Drawing for the job (mm, zero at the part's lowest x, y, z). A direction names the side the tool comes from. Give positions to 0.01 mm unless a question says otherwise; leave off trailing zeros. Order: outer loops, then holes, each group sorted by start corner. A loop starts at its lowest first (then second) coordinate and runs counter-clockwise, first axis right, second up. Notation, with made-up numbers: M -8.75,-21.75 L 24.25,-21.75 A21 ccw 24.25,3.25 Z; hole C 2.25,-22 d8. An arc over 180 degrees is marked long. Answer as a JSON object with one key per item and string values.
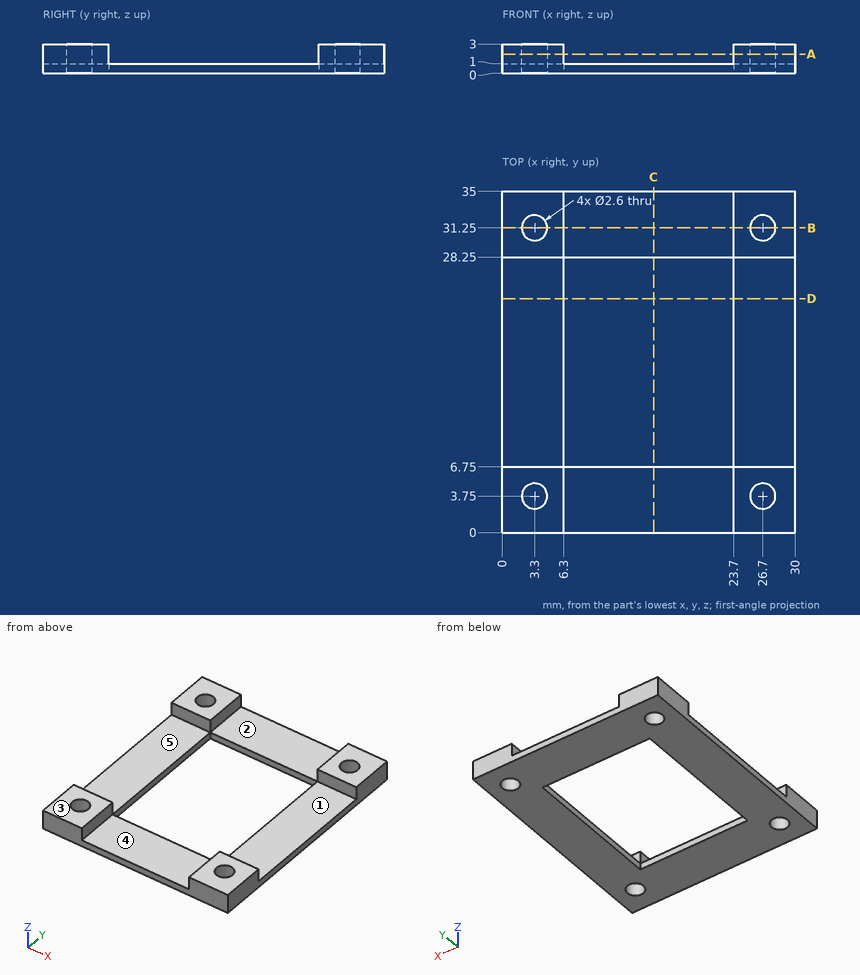
1. Pin check, flat tips, straight feed: P1, Ø4, axis at x = 5, y = 11.5, coming from the +Z side; P2, Ø2.5, axis at x = 3.3, y = 31.25, coming from the -Z side; P3, Ø1.1, axis at x = 11.5, z = 0.5, coming from the -Y side. Stop position of each tip, or through.
Worked answers:
{"P1": "stops at z = 1", "P2": "passes through", "P3": "stops at y = 0"}
2. Which spindle directions (+Z, -Z, +X, -X, +Y, -Y) get a long thin tool onto all of the face, cutting with end or side? Do the marked faces 1, 2 and 3. Say none if no direction does.
Worked answers:
{"face 1": "+Z, +X, -X", "face 2": "+Z, +Y, -Y", "face 3": "+Z, +X, -X, +Y, -Y"}
3. Cut at A-A on z = 1.95. Give the cut face in (x, y), plus the area to 3 significant figures.
Worked answers:
{"outline": "M 0,0 L 6.3,0 L 6.3,6.75 L 0,6.75 Z; M 0,28.25 L 6.3,28.25 L 6.3,35 L 0,35 Z; M 23.7,0 L 30,0 L 30,6.75 L 23.7,6.75 Z; M 23.7,28.25 L 30,28.25 L 30,35 L 23.7,35 Z; hole C 3.3,3.75 d2.6; hole C 3.3,31.25 d2.6; hole C 26.7,3.75 d2.6; hole C 26.7,31.25 d2.6", "area": "149 mm^2"}
4. Cut at B-B on y = 31.25. Give the cut face in (x, z), plus the area to 3 significant figures.
Worked answers:
{"outline": "M 0,0 L 2,0 L 2,3 L 0,3 Z; M 4.6,0 L 25.4,0 L 25.4,3 L 23.7,3 L 23.7,1 L 6.3,1 L 6.3,3 L 4.6,3 Z; M 28,0 L 30,0 L 30,3 L 28,3 Z", "area": "39.6 mm^2"}
5. Two-plate mould, pull along X, no slides. Class the marked faces 4 and 5: +X half, -X half, draft (parallel to the pull), parting line (faces both ways), or undercut.
Worked answers:
{"face 4": "undercut", "face 5": "draft"}
6. Probe line 1 along Y through (x, z) = (26.7, 0.85); line 2 along Y through (x, z) = (3.3, 2); line 3 along X through (y, z) = (5.5, 2.6). List the from-to ranges inside material, lowest first.
Worked answers:
{"line 1": "y = 0 to 2.45, 5.05 to 29.95, 32.55 to 35", "line 2": "y = 0 to 2.45, 5.05 to 6.75, 28.25 to 29.95, 32.55 to 35", "line 3": "x = 0 to 6.3, 23.7 to 30"}
7. Cut at D-D on y = 24. Give the cut face in (x, z), plus the area to 3 significant figures.
Worked answers:
{"outline": "M 0,0 L 6.3,0 L 6.3,1 L 0,1 Z; M 23.7,0 L 30,0 L 30,1 L 23.7,1 Z", "area": "12.6 mm^2"}
8. Cut at C-C on x = 15.5. Give the cut face in (y, z).
Worked answers:
{"outline": "M 0,0 L 6.75,0 L 6.75,1 L 0,1 Z; M 28.25,0 L 35,0 L 35,1 L 28.25,1 Z"}
